Autodesk Fusion 360 part; units mm, degrees
sketch "Sketch1" plane through (0, 0, 0) normal (0, 1, 0) x (1, 0, 0)
  arc A0 (0, -15) -> (0, 15) centre (0, 0) ccw
  line L0 (0, 0) -> (0, -15) construction
  line L1 (0, 0) -> (0, 15) construction
  line L2 (0, 15) -> (0, -15)
  circle A1 centre (7.5, 0) radius 5.5
  dimension "d1" = 180
  dimension "d2" = 11
  dimension "d10" = 7.5
extrude "Extrude1" add sketch "Sketch1" along normal blind 15
extrude "Extrude2" add sketch "Sketch1" along normal blind 25 contours A1
extrude "Extrude3" cut 1 faces at (7.6099, 25, -1.4661) along direction (0, -1, 0) blind 30
Work out the finished part from the listing and answer in its coordinate system (mm). Coordinates: 2 decimals unless noted, no trailing zeros. Write each loop counter-clockwise with the first axis right and the second up, starting at its lowest first coordinate (ties: lowest second). Pieces come first, ordered by that corner, then holes. Notation, with made-up numbers: (29, 34) - (86, 34) arc R5 ccw to (86, 42) - close; hole circle Ø10 at (14.25, -36.5). An arc over 180 degrees is marked (long way). Answer as a JSON object with one key per item and string values.
Q1. Consider L1, parallel to X at y = 11.25, z = 0; L2, parallel to Z at x = 7.5, y = 3; L3, parallel to Z at x = 11.75, y = 5.75. Determine where each line is inside the solid, lowest interval first. Write a range as from..to.
Results list:
{"L1": "x = 0..2, 13..15", "L2": "z = -12.99..-5.5, 5.5..12.99", "L3": "z = -9.32..-3.49, 3.49..9.32"}
Q2. Find section A-A (z = 0). Write down the section's boundary in (x, y).
Results list:
{"outline": "(0, 0) - (2, 0) - (2, 15) - (0, 15) - close; (13, 0) - (15, 0) - (15, 15) - (13, 15) - close"}
Q3. Find section C-C (y = 1). Write down the section's boundary in (x, z).
Results list:
{"outline": "(0, -15) arc R15 ccw to (0, 15) - close; hole circle Ø11 at (7.5, 0)"}
Q4. For a pull along X with two mould halves and no side action, classify faces 1 (the flat face through (0, 7, 0)), 2 (the flat face through (2, 15, -4)), 3 (the cylindrical face through (6.31, 7.6, 5.37)), 4 (the cylindrical face through (15, 7, 0)) as pulls with the +X half, pulls with the -X half, needs draft (parallel to the pull), parting line crosses it, or undercut.
Results list:
{"face 1": "pulls with the -X half", "face 2": "needs draft", "face 3": "undercut", "face 4": "pulls with the +X half"}
Q5. Find section B-B (x = 7.5). Write down the section's boundary in (y, z).
Results list:
{"outline": "(0, -12.99) - (15, -12.99) - (15, -5.5) - (0, -5.5) - close; (0, 5.5) - (15, 5.5) - (15, 12.99) - (0, 12.99) - close"}
Q6. Given pin 1 Ø5 at (x, y) = (12, 3) entering from -Z; pin 2 Ø5 at (x, y) = (4.5, 5.5) entering from -Z; pin 3 Ø8 at (x, y) = (11, 2) entering from -Z, each flat-ended and moving along its own axis, determine where each tip first touches the part or whether it passes through.
Results list:
{"pin 1": "stops at z = -11.61", "pin 2": "stops at z = -14.87", "pin 3": "stops at z = -13.27"}
Q7. Find section D-D (z = -9.5). Write down the section's boundary in (x, y), plus the area to 3 significant figures.
Results list:
{"outline": "(0, 0) - (11.61, 0) - (11.61, 15) - (0, 15) - close", "area": "174 mm^2"}
